from build123d import *

# Parameters (mm, degrees)
SKETCH1_R           = 18
SKETCH1_R_2         = 1.6
BOSS_EXTRUDE1_DEPTH = 3


with BuildPart() as part:
    # Sketch1 → Boss-Extrude1 (new body)
    with BuildSketch(Plane.XY):
        with BuildLine():
            Line((-63.5, -59), (63.5, -59))
            ThreePointArc((63.5, -59), (65.621320344, -58.121320344), (66.5, -56))
            Line((66.5, -56), (66.5, -28))
            Line((66.5, -28), (49.5, -28))
            Line((49.5, -28), (49.5, -15))
            Line((49.5, -15), (66.5, -15))
            Line((66.5, -15), (66.5, 3))
            Line((66.5, 3), (50.5, 3))
            Line((50.5, 3), (50.5, 38))
            Line((50.5, 38), (66.5, 38))
            Line((66.5, 38), (66.5, 56))
            ThreePointArc((66.5, 56), (65.621320344, 58.121320344), (63.5, 59))
            Line((63.5, 59), (-63.5, 59))
            ThreePointArc((-63.5, 59), (-65.621320344, 58.121320344), (-66.5, 56))
            Line((-66.5, 56), (-66.5, -56))
            ThreePointArc((-66.5, -56), (-65.621320344, -58.121320344), (-63.5, -59))
        make_face()
        with Locations((12.5, -2)):
            Circle(SKETCH1_R, mode=Mode.SUBTRACT)
        with Locations((-3.5, 14)):
            Circle(SKETCH1_R_2, mode=Mode.SUBTRACT)
        with Locations((28.5, 14)):
            Circle(SKETCH1_R_2, mode=Mode.SUBTRACT)
        with Locations((28.5, -18)):
            Circle(SKETCH1_R_2, mode=Mode.SUBTRACT)
        with Locations((-3.5, -18)):
            Circle(SKETCH1_R_2, mode=Mode.SUBTRACT)
        with Locations((-62.5, 55)):
            Circle(SKETCH1_R_2, mode=Mode.SUBTRACT)
        with Locations((62.5, 55)):
            Circle(SKETCH1_R_2, mode=Mode.SUBTRACT)
        with Locations((-62.5, -55)):
            Circle(SKETCH1_R_2, mode=Mode.SUBTRACT)
        with Locations((62.5, -55)):
            Circle(SKETCH1_R_2, mode=Mode.SUBTRACT)
        with BuildLine():
            Line((-55.75, 2.5), (-27.75, 2.5))
            ThreePointArc((-27.75, 2.5), (-25.25, 0), (-27.75, -2.5))
            Line((-27.75, -2.5), (-55.75, -2.5))
            ThreePointArc((-55.75, -2.5), (-58.25, 0), (-55.75, 2.5))
        make_face(mode=Mode.SUBTRACT)
        with BuildLine():
            Line((-55.75, 12.5), (-27.75, 12.5))
            ThreePointArc((-27.75, 12.5), (-25.25, 10), (-27.75, 7.5))
            Line((-27.75, 7.5), (-55.75, 7.5))
            ThreePointArc((-55.75, 7.5), (-58.25, 10), (-55.75, 12.5))
        make_face(mode=Mode.SUBTRACT)
        with BuildLine():
            Line((-55.75, 22.5), (-27.75, 22.5))
            ThreePointArc((-27.75, 22.5), (-25.25, 20), (-27.75, 17.5))
            Line((-27.75, 17.5), (-55.75, 17.5))
            ThreePointArc((-55.75, 17.5), (-58.25, 20), (-55.75, 22.5))
        make_face(mode=Mode.SUBTRACT)
        with BuildLine():
            Line((-55.75, 32.5), (-27.75, 32.5))
            ThreePointArc((-27.75, 32.5), (-25.25, 30), (-27.75, 27.5))
            Line((-27.75, 27.5), (-55.75, 27.5))
            ThreePointArc((-55.75, 27.5), (-58.25, 30), (-55.75, 32.5))
        make_face(mode=Mode.SUBTRACT)
        with BuildLine():
            Line((-55.75, 42.5), (-27.75, 42.5))
            ThreePointArc((-27.75, 42.5), (-25.25, 40), (-27.75, 37.5))
            Line((-27.75, 37.5), (-55.75, 37.5))
            ThreePointArc((-55.75, 37.5), (-58.25, 40), (-55.75, 42.5))
        make_face(mode=Mode.SUBTRACT)
        with BuildLine():
            Line((-55.75, -37.5), (-27.75, -37.5))
            ThreePointArc((-27.75, -37.5), (-25.25, -40), (-27.75, -42.5))
            Line((-27.75, -42.5), (-55.75, -42.5))
            ThreePointArc((-55.75, -42.5), (-58.25, -40), (-55.75, -37.5))
        make_face(mode=Mode.SUBTRACT)
        with BuildLine():
            Line((-55.75, -27.5), (-27.75, -27.5))
            ThreePointArc((-27.75, -27.5), (-25.25, -30), (-27.75, -32.5))
            Line((-27.75, -32.5), (-55.75, -32.5))
            ThreePointArc((-55.75, -32.5), (-58.25, -30), (-55.75, -27.5))
        make_face(mode=Mode.SUBTRACT)
        with BuildLine():
            Line((-55.75, -17.5), (-27.75, -17.5))
            ThreePointArc((-27.75, -17.5), (-25.25, -20), (-27.75, -22.5))
            Line((-27.75, -22.5), (-55.75, -22.5))
            ThreePointArc((-55.75, -22.5), (-58.25, -20), (-55.75, -17.5))
        make_face(mode=Mode.SUBTRACT)
        with BuildLine():
            Line((-55.75, -7.5), (-27.75, -7.5))
            ThreePointArc((-27.75, -7.5), (-25.25, -10), (-27.75, -12.5))
            Line((-27.75, -12.5), (-55.75, -12.5))
            ThreePointArc((-55.75, -12.5), (-58.25, -10), (-55.75, -7.5))
        make_face(mode=Mode.SUBTRACT)
    extrude(amount=BOSS_EXTRUDE1_DEPTH)


solid = part.part
Can you work these out from the model? Positions are in its coordinate system, mm. A direction names the side the tool comes from. Coordinates: 2 decimals unless noted, no trailing zeros. Order: outer loops, then holes, each group sorted by start corner. A loop starts at its lowest first (then second) coordinate and runs counter-clockwise, first axis right, second up. Notation, with made-up numbers: (27.25, 71.25) -> (36.25, 71.25) arc R24 cw to (36.25, 91.25) -> close; hole circle Ø2 at (54, 46). An arc over 180 degrees is marked (long way). Use one line per item in the form item = value.
Q1. We'd pull the mould along X, two halves only. Please class faces 1 (the face through (66.5, 47, 1)), 2 (the face through (58, -15, 1)), 3 (the face through (-25.25, 40.05, 1.48)): released by +X, released by -X, zero draft, split by the parting line, or undercut.
From the geometry:
face_1 = released by +X
face_2 = zero draft
face_3 = undercut
Q2. Imagine slicing it at C-C, the plane y = 10. List the corners of the cut face in (x, z) for me.
From the geometry:
outline = (-66.5, 0) -> (-58.25, 0) -> (-58.25, 3) -> (-66.5, 3) -> close; (-25.25, 0) -> (-0.92, 0) -> (-0.92, 3) -> (-25.25, 3) -> close; (25.92, 0) -> (50.5, 0) -> (50.5, 3) -> (25.92, 3) -> close
Q3. Imagine slicing it at B-B, the plane y = 30. List the corners of the cut face in (x, z) for me.
From the geometry:
outline = (-66.5, 0) -> (-58.25, 0) -> (-58.25, 3) -> (-66.5, 3) -> close; (-25.25, 0) -> (50.5, 0) -> (50.5, 3) -> (-25.25, 3) -> close
Q4. Which directions (+Z, -Z, +X, -X, +Y, -Y) give clear straight access to the entire face, cutting with the end or side of a thin tool? Please do faces 4 (the face through (-1, 14, 0)), 5 (the face through (-42, 22.5, 1)), 6 (the face through (58, -28, 1)).
From the geometry:
face_4 = -Z, +X, -X, +Y, -Y
face_5 = +Z, -Z
face_6 = +Z, -Z, +X
Q5. Imagine slicing it at D-D, the plane x = -3.5. List the corners of the cut face in (y, z) for me, then the cut area to 3 significant figures.
From the geometry:
outline = (-59, 0) -> (-19.6, 0) -> (-19.6, 3) -> (-59, 3) -> close; (-16.4, 0) -> (-10.25, 0) -> (-10.25, 3) -> (-16.4, 3) -> close; (6.25, 0) -> (12.4, 0) -> (12.4, 3) -> (6.25, 3) -> close; (15.6, 0) -> (59, 0) -> (59, 3) -> (15.6, 3) -> close
area = 285 mm²
Q6. I need wall thicknesses on L1, parallel to Y at x = -62.5, z = 2.35; L2, parallel to Y at x = 62.5, z = 1.75; L3, parallel to Y at x = 12.5, z = 1.2. Which ranges of each line are inside material? Lowest first, please.
From the geometry:
L1 = -59 to -56.6, -53.4 to 53.4, 56.6 to 59
L2 = -59 to -56.6, -53.4 to -28, -15 to 3, 38 to 53.4, 56.6 to 59
L3 = -59 to -20, 16 to 59
Q7. Will this pin go through, and if not, where does the flat tip stop? P1, Ø2, axis at x = -29, y = 5.5, coming from the -Z side.
From the geometry:
P1 = 0
Q8. Imagine slicing it at A-A, the plane x = 52. List the corners of the cut face in (y, z) for me, then the cut area to 3 significant figures.
From the geometry:
outline = (-59, 0) -> (-28, 0) -> (-28, 3) -> (-59, 3) -> close; (-15, 0) -> (3, 0) -> (3, 3) -> (-15, 3) -> close; (38, 0) -> (59, 0) -> (59, 3) -> (38, 3) -> close
area = 210 mm²
